Build history of the part. All positions in model axes, mm. A direction names the side the tool comes from. Coordinates: 2 decimals unless noted, no trailing zeros. Loops run counter-clockwise (first coordinate to the right, second up) from the corner with the lowest first, then second, coordinate; pieces in that order, holes last.
Item 1: Mould opens along X. For faces 1 (the face through (-7, 0, 44)), 2 (the face through (10, 2, 44)), 3 (the face through (0, 2, 75)), 4 (the face through (-1.08, 2.46, 94.88)) say: released by +X, released by -X, zero draft, split by the parting line, or undercut.
Item 2: 3-axis set-ups, long thin cutter, end or side, ignore diameter. For faces 5 (the face through (5, 2, 45)), 6 (the face through (0, 2, 100)): which of +Z, -Z, +X, -X, +Y, -Y reach the whole face in a straight line?
Item 3: Drill centre lines: line 1 along Z through (x, y) = (0, 1.1); line 2 along X through (y, z) = (2.25, 0); line 3 along Z through (x, y) = (3.5, 3.3). Where is each one in solid material? Low to high.
Item 4: Cut at B-B (x = 0). List the corners of the cut face in (y, z).
Item 5: Cut at C-C (y = 1.3). List the corners of the cut face in (x, z), and give its area (3 significant figures).
Item 6: Cut at D-D (z = 25). List the corners of the cut face in (x, y), and give its area (3 significant figures).
Item 7: Cut at A-A (z = 86.5). List the corners of the cut face in (x, y), and give its area (3 significant figures).
Item 8: Flat gauge pin, fed straight in: pin 1 (6 mm diameter, centred on x = 0, z = 90, fed in from +Y). Where does the tip first touch, or does it go through?
from build123d import *

# Parameters (mm, degrees)
SKETCH1_R           = 5
BOSS_EXTRUDE1_DEPTH = 5


with BuildPart() as part:
    # Sketch1 → Boss-Extrude1 (new body)
    with BuildSketch(Plane(origin=(0, 0, 0), x_dir=(1, 0, 0), z_dir=(0, 1, 0))):
        with BuildLine():
            Line((10, 0), (10, -90))
            ThreePointArc((10, -90), (0, -100), (-10, -90))
            Line((-10, -90), (-10, 0))
            ThreePointArc((-10, 0), (0, 10), (10, 0))
        make_face()
        Circle(SKETCH1_R, mode=Mode.SUBTRACT)
        with Locations((0, -90)):
            Circle(SKETCH1_R, mode=Mode.SUBTRACT)
        with BuildLine():
            Line((5, -20), (5, -70))
            ThreePointArc((5, -70), (0, -75), (-5, -70))
            Line((-5, -70), (-5, -20))
            ThreePointArc((-5, -20), (0, -15), (5, -20))
        make_face(mode=Mode.SUBTRACT)
    extrude(amount=BOSS_EXTRUDE1_DEPTH)


solid = part.part
Filled sheet:
1. face 1: zero draft
1. face 2: released by +X
1. face 3: undercut
1. face 4: undercut
2. face 5: +Y, -Y
2. face 6: +Z, +Y, -Y
3. line 1: z = -10 to -5, 5 to 15, 75 to 85, 95 to 100
3. line 2: x = -10 to -5, 5 to 10
3. line 3: z = -9.37 to -3.57, 3.57 to 16.43, 73.57 to 86.43, 93.57 to 99.37
4. outline: (0, -10) - (5, -10) - (5, -5) - (0, -5) - close; (0, 5) - (5, 5) - (5, 15) - (0, 15) - close; (0, 75) - (5, 75) - (5, 85) - (0, 85) - close; (0, 95) - (5, 95) - (5, 100) - (0, 100) - close
5. outline: (-10, 0) arc R10 ccw to (10, 0) - (10, 90) arc R10 ccw to (-10, 90) - close; hole circle Ø10 at (0, 0); hole (-5, 20) arc R5 ccw to (5, 20) - (5, 70) arc R5 ccw to (-5, 70) - close; hole circle Ø10 at (0, 90)
5. area: 1,380 mm2
6. outline: (-10, 0) - (-5, 0) - (-5, 5) - (-10, 5) - close; (5, 0) - (10, 0) - (10, 5) - (5, 5) - close
6. area: 50.0 mm2
7. outline: (-10, 0) - (-3.57, 0) - (-3.57, 5) - (-10, 5) - close; (3.57, 0) - (10, 0) - (10, 5) - (3.57, 5) - close
7. area: 64.3 mm2
8. pin 1: passes through
